```python
from build123d import *

# Parameters (mm, degrees)
F0_W     = 500
F0_H     = 500
F0_W_2   = 460
F0_H_2   = 460
F1_DEPTH = 450
F2_W     = 20
F2_H     = 460
F3_DEPTH = 455


with BuildPart() as f1:
    # F0 (on Front) → F1 (new body)
    with BuildSketch(Plane.XZ):
        Rectangle(F0_W, F0_H)
        Rectangle(F0_W_2, F0_H_2, mode=Mode.SUBTRACT)
    extrude(amount=F1_DEPTH)

    # F2 (on face) → F3 (join)
    with BuildSketch(Plane.YZ.offset(-230)):
        with Locations((-435, 0)):
            Rectangle(F2_W, F2_H)
    extrude(amount=F3_DEPTH)

    # F4 (on Top) → F5 (revolve)
    with BuildSketch(Plane.XY):
        with BuildLine():
            Line((166.631432, -424.459219), (157.49906, -426.544428))
            Line((157.49906, -426.544428), (157.49906, -511.243738))
            ThreePointArc((157.49906, -511.243738), (174.167415, -507.082896), (186.924866, -495.576632))
            ThreePointArc((186.924866, -495.576632), (172.751683, -483.986573), (166.631432, -466.731107))
            Line((166.631432, -466.731107), (166.631432, -424.459219))
        make_face()
    revolve(axis=Axis((157.49906, -468.894083, 0), (0, -1, 0)))


solid = f1.part
```
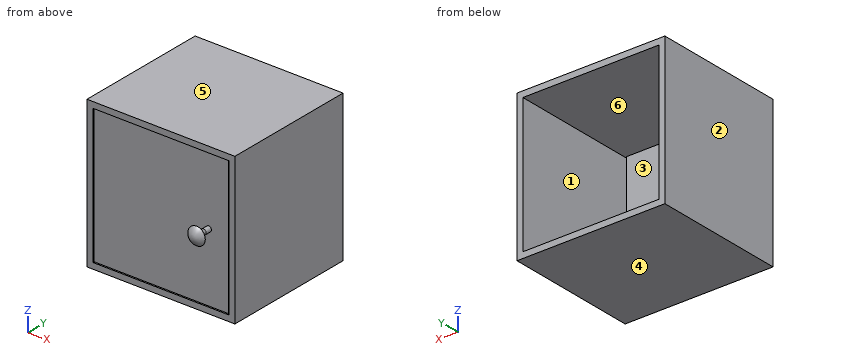
Verification items for the finished model (mm, model axes). Face numbers are marked on the shaded views. A direction names the side the tool comes from. Coordinates: 2 decimals unless noted, no trailing zeros. Order: outer loops, then holes, each group sorted by start corner. A loop starts at its lowest first (then second) coordinate and runs counter-clockwise, first axis right, second up. Notation, with made-up numbers: (68, 48.5) -> (111, 48.5) arc R30 cw to (111, 87.5) -> close; hole circle Ø4 at (4.25, -33). An arc over 180 degrees is marked (long way). Put each result on its own line as item: value. Start each with the question number.
1) Cross-section at B-B (x = -74). Enter the section's corners in (y, z).
2) Go/stop test with flat-tipped pins: pin 1 (8 mm diameter, centred on x = 88, z = -113, fed in from -Y); pin 2 (4 mm diameter, centred on x = 160, z = 0.5, fed in from +Y). Record where each tip stops, or that it passes through.
3) Material ranges on L1, parallel to X at y = -257.5, z = -142; L2, parallel to Y at x = 200, z = -47.5, recorded low to high.
4) Cross-section at C-C (y = -252). Enter the section's corners in (x, z).
5) Tool access check on the marked faces 1, 2 and 3. Record the directions out of +Z, -Z, +X, -X, +Y, -Y that give a thin tool (end or side, any length) a straight path to the whole face; none if there is none.
6) Cross-section at A-A (z = 199). Enter the section's corners in (x, y), plus the area to 3 significant figures.
7) Release check for a two-part mould opening along Z. For the marked faces 4, 5 and 6 record: pulls with the +Z half, pulls with the -Z half, needs draft (parallel to the pull), parting line crosses it, or undercut.
Geometry check:
1. outline: (-450, -250) -> (0, -250) -> (0, -230) -> (-425, -230) -> (-425, 230) -> (0, 230) -> (0, 250) -> (-450, 250) -> (-450, 230) -> (-445, 230) -> (-445, -230) -> (-450, -230) -> close
2. pin 1: stops at y = -445
2. pin 2: stops at y = -425
3. L1: x = -250 to -230, 230 to 250
3. L2: y = -445 to -425
4. outline: (-250, -250) -> (250, -250) -> (250, 250) -> (-250, 250) -> close; hole (-230, -230) -> (230, -230) -> (230, 230) -> (-230, 230) -> close
5. face 1: +Y, -Y
5. face 2: +Z, -Z, -X, +Y, -Y
5. face 3: +Y
6. outline: (-250, -450) -> (-230, -450) -> (-230, -445) -> (225, -445) -> (225, -425) -> (-230, -425) -> (-230, 0) -> (-250, 0) -> close; (230, -450) -> (250, -450) -> (250, 0) -> (230, 0) -> close
6. area: 27,100 mm^2
7. face 4: pulls with the -Z half
7. face 5: pulls with the +Z half
7. face 6: undercut
